```python
from build123d import *

# Parameters (mm, degrees)
CROQUIS1_W              = 340.36
CROQUIS1_H              = 203.2
SALIENTE_EXTRUIR1_DEPTH = 5.08
CROQUIS2_W              = 12.7
CROQUIS2_H              = 91.44
SALIENTE_EXTRUIR2_DEPTH = 1.27
CROQUIS3_R              = 4.191
CORTAR_EXTRUIR1_DEPTH   = 10
REDONDEO1_R             = 5.08


with BuildPart() as part:
    # Croquis1 → Saliente-Extruir1 (new body)
    with BuildSketch(Plane(origin=(0, 0, 0), x_dir=(1, 0, 0), z_dir=(0, 1, 0))):
        Rectangle(CROQUIS1_W, CROQUIS1_H)
    extrude(amount=SALIENTE_EXTRUIR1_DEPTH)

    # Croquis2 → Saliente-Extruir2 (add)
    with BuildSketch(Plane(origin=(0, 5.08, 0), x_dir=(1, 0, 0), z_dir=(0, 1, 0))):
        with Locations((-143.51, 48.26)):
            Rectangle(CROQUIS2_W, CROQUIS2_H)
        with Locations((-126.626470588, 48.26)):
            Rectangle(CROQUIS2_W, CROQUIS2_H)
        with Locations((-109.742941176, 48.26)):
            Rectangle(CROQUIS2_W, CROQUIS2_H)
        with Locations((-92.859411765, 48.26)):
            Rectangle(CROQUIS2_W, CROQUIS2_H)
        with Locations((-75.975882353, 48.26)):
            Rectangle(CROQUIS2_W, CROQUIS2_H)
        with Locations((-59.092352941, 48.26)):
            Rectangle(CROQUIS2_W, CROQUIS2_H)
        with Locations((-42.208823529, 48.26)):
            Rectangle(CROQUIS2_W, CROQUIS2_H)
        with Locations((-25.325294118, 48.26)):
            Rectangle(CROQUIS2_W, CROQUIS2_H)
        with Locations((-8.441764706, 48.26)):
            Rectangle(CROQUIS2_W, CROQUIS2_H)
        with Locations((8.441764706, 48.26)):
            Rectangle(CROQUIS2_W, CROQUIS2_H)
        with Locations((25.325294118, 48.26)):
            Rectangle(CROQUIS2_W, CROQUIS2_H)
        with Locations((42.208823529, 48.26)):
            Rectangle(CROQUIS2_W, CROQUIS2_H)
        with Locations((59.092352941, 48.26)):
            Rectangle(CROQUIS2_W, CROQUIS2_H)
        with Locations((75.975882353, 48.26)):
            Rectangle(CROQUIS2_W, CROQUIS2_H)
        with Locations((92.859411765, 48.26)):
            Rectangle(CROQUIS2_W, CROQUIS2_H)
        with Locations((109.742941176, 48.26)):
            Rectangle(CROQUIS2_W, CROQUIS2_H)
        with Locations((126.626470588, 48.26)):
            Rectangle(CROQUIS2_W, CROQUIS2_H)
        with Locations((143.51, 48.26)):
            Rectangle(CROQUIS2_W, CROQUIS2_H)
        with Locations((143.51, -48.26)):
            Rectangle(CROQUIS2_W, CROQUIS2_H)
        with Locations((126.626470588, -48.26)):
            Rectangle(CROQUIS2_W, CROQUIS2_H)
        with Locations((109.742941176, -48.26)):
            Rectangle(CROQUIS2_W, CROQUIS2_H)
        with Locations((92.859411765, -48.26)):
            Rectangle(CROQUIS2_W, CROQUIS2_H)
        with Locations((75.975882353, -48.26)):
            Rectangle(CROQUIS2_W, CROQUIS2_H)
        with Locations((59.092352941, -48.26)):
            Rectangle(CROQUIS2_W, CROQUIS2_H)
        with Locations((42.208823529, -48.26)):
            Rectangle(CROQUIS2_W, CROQUIS2_H)
        with Locations((25.325294118, -48.26)):
            Rectangle(CROQUIS2_W, CROQUIS2_H)
        with Locations((8.441764706, -48.26)):
            Rectangle(CROQUIS2_W, CROQUIS2_H)
        with Locations((-8.441764706, -48.26)):
            Rectangle(CROQUIS2_W, CROQUIS2_H)
        with Locations((-25.325294118, -48.26)):
            Rectangle(CROQUIS2_W, CROQUIS2_H)
        with Locations((-42.208823529, -48.26)):
            Rectangle(CROQUIS2_W, CROQUIS2_H)
        with Locations((-59.092352941, -48.26)):
            Rectangle(CROQUIS2_W, CROQUIS2_H)
        with Locations((-75.975882353, -48.26)):
            Rectangle(CROQUIS2_W, CROQUIS2_H)
        with Locations((-92.859411765, -48.26)):
            Rectangle(CROQUIS2_W, CROQUIS2_H)
        with Locations((-109.742941176, -48.26)):
            Rectangle(CROQUIS2_W, CROQUIS2_H)
        with Locations((-126.626470588, -48.26)):
            Rectangle(CROQUIS2_W, CROQUIS2_H)
        with Locations((-143.51, -48.26)):
            Rectangle(CROQUIS2_W, CROQUIS2_H)
    extrude(amount=SALIENTE_EXTRUIR2_DEPTH)

    # Croquis3 → Cortar-Extruir1 (cut)
    with BuildSketch(Plane(origin=(0, 5.08, 0), x_dir=(1, 0, 0), z_dir=(0, 1, 0))):
        with Locations(Location((-160.909, -82.169, 0), (0, 0, 270))):
            Circle(CROQUIS3_R)
        with Locations(Location((160.909, -82.169, 0), (0, 0, 270))):
            Circle(CROQUIS3_R)
    extrude(amount=-CORTAR_EXTRUIR1_DEPTH, mode=Mode.SUBTRACT)

    # Redondeo1
    redondeo1_edges = [part.edges().sort_by_distance(p)[0] for p in [
        (-170.18, 2.54, -101.6),
        (170.18, 2.54, -101.6),
        (170.18, 2.54, 101.6),
        (-170.18, 2.54, 101.6),
    ]]
    fillet(redondeo1_edges, radius=REDONDEO1_R)


solid = part.part
```
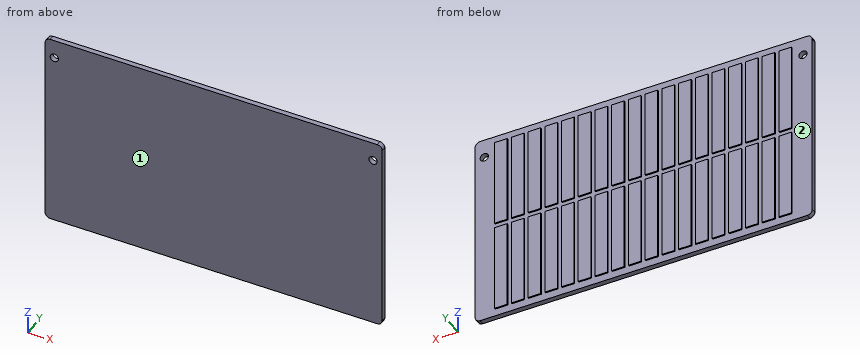
Work out the finished part from the listing and answer in its coordinate system (mm). Face numbers are marked on the shaded views. Give positions to 0.01 mm unless a question says otherwise; leave off trailing zeros. Loops run counter-clockwise (first coordinate to the right, second up) from the corner with the lowest first, then second, coordinate; pieces in that order, holes last. Notation, with made-up numbers: (43.25, -1) - (85.25, -1) arc R18 ccw to (85.25, 29) - close; hole circle Ø2 at (45, 57.25). An arc over 180 degrees is marked (long way). Use CSV: the item, a comma, the result in double quotes. Start each with the question number.
(1) Determine the mould class of the marked faces 1 and 2 for opening direction X: released by +X, released by -X, zero draft, split by the parting line, or undercut.
(2) Find the intervals of material crossed by L1, parallel to Y at x = 152.5, z = -80.5, in increasing order.
(3) Each of these flat-tipped pins is pushed along its axis until it touches: pin 1 (0.6 mm diameter, centred on x = -23.5, y = 5.5, fed in from +Z); pin 2 (0.6 mm diameter, centred on y = 5.5, z = -61.5, fed in from -X); pin 3 (1 mm diameter, centred on x = -77.5, y = 6, fed in from -Z). Where does it stop, or does it pass through?
(4) Find section A-A, the plane x = 10. Determine the outline of the cut face in (y, z), plus the area to 3 significant figures.
Results found:
1,face 1,"zero draft"
1,face 2,"undercut"
2,L1,"0 to 5.08"
3,pin 1,"z = 93.98"
3,pin 2,"x = -149.86"
3,pin 3,"z = -93.98"
4,outline,"(0, -101.6) - (5.08, -101.6) - (5.08, -93.98) - (6.35, -93.98) - (6.35, -2.54) - (5.08, -2.54) - (5.08, 2.54) - (6.35, 2.54) - (6.35, 93.98) - (5.08, 93.98) - (5.08, 101.6) - (0, 101.6) - close"
4,area,"1,260 mm^2"
